```python
from build123d import *

# Parameters (mm, degrees)
SKETCH3_W           = 232.55
SKETCH3_H           = 63.5
SKETCH3_R           = 2.778125
SKETCH3_R_2         = 23.495
BOSS_EXTRUDE1_DEPTH = 10
CIRPATTERN1_COUNT   = 7
FILLET1_R           = 63.5
SKETCH4_R           = 3.25
CUT_EXTRUDE1_DEPTH  = 11


with BuildPart() as part:
    # Sketch3 → Boss-Extrude1 (new body)
    with BuildSketch(Plane(origin=(0, 0, 0), x_dir=(1, 0, 0), z_dir=(0, 1, 0))):
        with Locations((116.275, 0)):
            Rectangle(SKETCH3_W, SKETCH3_H)
        with Locations((159.525, 22.225)):
            Circle(SKETCH3_R, mode=Mode.SUBTRACT)
        with Locations((159.525, -22.225)):
            Circle(SKETCH3_R, mode=Mode.SUBTRACT)
        with Locations((200.8, 0)):
            Circle(SKETCH3_R_2, mode=Mode.SUBTRACT)
    boss_extrude1 = extrude(amount=BOSS_EXTRUDE1_DEPTH)

    # CirPattern1: Boss-Extrude1 ×7 about axis
    cirpattern1_axis = Axis((0, 0, 0), (0, 1, 0))
    for i in range(1, CIRPATTERN1_COUNT):
        add(boss_extrude1.rotate(cirpattern1_axis, i * 360 / CIRPATTERN1_COUNT))

    # Fillet1
    fillet1_edges = [part.edges().sort_by_distance(p)[0] for p in [
        (65.929554341, 5, 31.75),
        (65.929554341, 5, -31.75),
        (16.283255204, 5, 71.341602418),
        (-45.624667219, 5, 57.211523112),
        (-73.176284653, 5, 0),
        (-45.624667219, 5, -57.211523112),
        (16.283255204, 5, -71.341602418),
    ]]
    fillet(fillet1_edges, radius=FILLET1_R)

    # Sketch4 → Cut-Extrude1 (cut, through all)
    with BuildSketch(Plane(origin=(0, 0, 0), x_dir=(1, 0, 0), z_dir=(0, 1, 0))):
        with Locations((75, 75)):
            Circle(SKETCH4_R)
        with Locations((75, -75)):
            Circle(SKETCH4_R)
        with Locations((-75, -75)):
            Circle(SKETCH4_R)
        with Locations((-75, 75)):
            Circle(SKETCH4_R)
        Circle(SKETCH4_R)
    extrude(amount=CUT_EXTRUDE1_DEPTH, mode=Mode.SUBTRACT)


solid = part.part
```
The listing builds one solid part. Answer for the finished solid, in the listing's coordinates (mm). A direction names the side the tool comes from. Coordinates: 2 decimals unless noted, no trailing zeros. Return JSON: item names as keys, results as strings. Group by question number.
1. Which of the six approach directions +Z, -Z, +X, -X, +Y, -Y give full straight-line access (tool end or side, diameter ignored) to faces 1 (the flat face through (158.827, 4.93, 148.24)), 2 (the flat face through (109.18, 4.93, -187.83)), 3 (the flat face through (109.18, 4.93, 187.83))?
2. Determine the mould class of faces 4 (the flat face through (215, 5, -31.75)), 5 (the flat face through (-52.18, 4.93, 226.62)), 6 (the flat face through (3.5, 10, -0.9)), 7 (the cylindrical face through (-96.507, 5.07, 122.616)) for opening direction Z: released by +Z, released by -Z, zero draft, split by the parting line, or undercut.
3. Given pin 1 (1 mm diameter, centred on y = 4.5, z = 18.5, fed in from -X); pin 2 (1 mm diameter, centred on x = -5, y = 7, fed in from +Z); pin 3 (1.5 mm diameter, centred on y = 2, z = -158, fed in from +X), each flat-ended and moving along its own axis, determine where each tip first touches the part or whether it passes through.
4. Straight lines are drawn through the part: L1, parallel to Z at x = -198.5, y = 4.5; L2, parallel to X at y = 6.75, z = 136.5; L3, parallel to X at y = 9.5, z = -198.5. For each, find the intervals that lie inside material, in ascending order.
5. A cutting plane is placed at A-A, the plane y = 4.75. Give the number of separate pieces and of enclosed holes in the cut face, plus the area to 3 significant figures.
Ans:
{
 "1": {"face 1": "+X, +Y, -Y", "face 2": "-Z, +Y, -Y", "face 3": "+Z, +Y, -Y"},
 "2": {"face 4": "released by -Z", "face 5": "released by +Z", "face 6": "zero draft", "face 7": "undercut"},
 "3": {"pin 1": "x = -158.94", "pin 2": "z = 181.19", "pin 3": "x = 167.21"},
 "4": {"L1": "-123.78 to -102.7, -71.54 to -60.35, 60.35 to 71.54, 102.7 to 123.78", "L2": "-83.98 to 80.24, 83.93 to 113.7, 136.69 to 149.46", "L3": "-77.87 to -68.02, -21.35 to -12.72, 117.69 to 124.07"},
 "5": {"separate pieces": "1", "enclosed holes": "26", "area": "103,000 mm²"}
}
